Part model, mm, in its own coordinate system. A direction names the side the tool comes from. Give positions to 0.01 mm unless a question says otherwise; leave off trailing zeros. Loops run counter-clockwise (first coordinate to the right, second up) from the corner with the lowest first, then second, coordinate; pieces in that order, holes last. Notation, with made-up numbers: (22, -3.75) -> (37, -3.75) arc R20 cw to (37, 13.25) -> close; hole circle Ø1 at (7.5, 22). An arc over 180 degrees is marked (long way). One line per question, with ' | ' between items.
```python
from build123d import *

# Parameters (mm, degrees)
SKETCH_1_R      = 2
SKETCH_1_R_2    = 1
EXTRUDE_1_DEPTH = 100
SKETCH_2_W      = 0.5
SKETCH_2_H      = 3
SKETCH_4_W      = 0.5
SKETCH_4_H      = 50


with BuildPart() as part:
    # Эскиз1 → Бобышка-Вытянуть1 (new body)
    with BuildSketch(Plane(origin=(0, 0, 0), x_dir=(1, 0, 0), z_dir=(0, 1, 0))):
        Circle(SKETCH_1_R)
        Circle(SKETCH_1_R_2, mode=Mode.SUBTRACT)
    extrude(amount=EXTRUDE_1_DEPTH)

    # Эскиз2 → Вырез-Повернуть1 (revolve, cut)
    with BuildSketch(Plane.XY):
        with Locations((1.75, 1.5)):
            Rectangle(SKETCH_2_W, SKETCH_2_H)
        with Locations((1.75, 8.5)):
            Rectangle(SKETCH_2_W, SKETCH_2_H)
    revolve(axis=Axis((0, 0, 0), (0, 1, 0)), mode=Mode.SUBTRACT)

    # Эскиз4 → Вырез-Повернуть2 (revolve, cut)
    with BuildSketch(Plane.XY):
        with Locations((1.75, 75)):
            Rectangle(SKETCH_4_W, SKETCH_4_H)
    revolve(axis=Axis((0, 0, 0), (0, 1, 0)), mode=Mode.SUBTRACT)


solid = part.part
```
1) Pull direction X, two halves, no side cores. Call faces 1 (the cylindrical face through (0, 30, 2)), 2 (the cylindrical face through (0, 49, 1)): pulls with the +X half, pulls with the -X half, needs draft (parallel to the pull), parting line crosses it, or undercut.
Found:
face 1: parting line crosses it | face 2: undercut
2) Saw through at B-B (x = 0). Give the cut face in (y, z).
Found:
outline: (0, -1.5) -> (3, -1.5) -> (3, -2) -> (7, -2) -> (7, -1.5) -> (10, -1.5) -> (10, -2) -> (50, -2) -> (50, -1.5) -> (100, -1.5) -> (100, -1) -> (0, -1) -> close; (0, 1) -> (100, 1) -> (100, 1.5) -> (50, 1.5) -> (50, 2) -> (10, 2) -> (10, 1.5) -> (7, 1.5) -> (7, 2) -> (3, 2) -> (3, 1.5) -> (0, 1.5) -> close
3) Drill centre lines: line 1 (X direction, y = 68, z = 0); line 2 (Y direction, x = -0.65, z = -1.4); line 3 (X direction, y = 23.5, z = 0). Where is each one in solid material? Low to high.
Found:
line 1: -1.5 to -1, 1 to 1.5 | line 2: 3 to 7, 10 to 50 | line 3: -2 to -1, 1 to 2
4) Saw through at C-C (y = 56). Give the cut face in (x, z), and give its area (3 significant figures).
Found:
outline: circle Ø3 at (0, 0); hole circle Ø2 at (0, 0) | area: 3.93 mm2
5) Saw through at D-D (y = 37). Give the cut face in (x, z), and give its area (3 significant figures).
Found:
outline: circle Ø4 at (0, 0); hole circle Ø2 at (0, 0) | area: 9.42 mm2
6) Tool access for faces 3 (the cylindrical face through (0, 5, 2)), 4 (the cylindrical face through (-1.5, 8.52, -0.07)), 5 (the cylindrical face through (-1.5, 1.52, -0.07)), 6 (the cylindrical face through (-1.5, 75.35, -0.07)): list every direction of +Z, -Z, +X, -X, +Y, -Y with a clear straight run to the whole face (end or side of a thin tool).
Found:
face 3: +Y, -Y | face 4: none | face 5: -Y | face 6: +Y
7) Saw through at A-A (z = 0). Give the cut face in (x, y), and give its area (3 significant figures).
Found:
outline: (-2, 3) -> (-1.5, 3) -> (-1.5, 0) -> (-1, 0) -> (-1, 100) -> (-1.5, 100) -> (-1.5, 50) -> (-2, 50) -> (-2, 10) -> (-1.5, 10) -> (-1.5, 7) -> (-2, 7) -> close; (1, 0) -> (1.5, 0) -> (1.5, 3) -> (2, 3) -> (2, 7) -> (1.5, 7) -> (1.5, 10) -> (2, 10) -> (2, 50) -> (1.5, 50) -> (1.5, 100) -> (1, 100) -> close | area: 144 mm2
